Can you work these out from the model? Positions are in its coordinate system, mm. A direction names the side the tool comes from. Round coordinates to 2 decimals unless told otherwise and drop trailing zeros. Loops run counter-clockwise (first coordinate to the right, second up) from the corner with the lowest first, then second, coordinate; pieces in that order, holes last.
(1) I want a section at A-A on x = 0. Write out the boundary of the cut face in (y, z).
(2) I want a section at B-B on y = 12.5. Write out the boundary of the cut face in (x, z), plus the area to 3 significant figures.
(3) If I drill on line 1 along Y through (x, z) = (4.15, 0); line 2 along X through (y, z) = (8, 0); line 3 along X through (y, z) = (-12, -2.75), over which ranges is the centre line in solid material (lowest first)?
(4) Will these pins go through, and if not, where does the flat tip stop? pin 1 Ø0.8 at (x, z) = (0.5, -4) entering from -Y; pin 2 Ø5 at (x, z) = (3.5, 1.5) entering from +Y; pin 3 Ø2.5 at (y, z) = (-1, -2) entering from -X; pin 4 Ø1.2 at (x, z) = (-0.5, -4) entering from +Y.
(5) Thinking about a two-plate mould opening in Y: for faces 6 (the face through (-4, 12, 0)), 7 (the face through (0, -2, 2.5)), 8 (the face through (0, 2.964, 4)), which applies, released by +Y, released by -Y, zero draft, split by the parting line, or undercut?
(6) I want a section at C-C on z = -3. Write out the boundary of the cut face in (x, y), plus the area to 3 significant figures.
(7) Which directions (+Z, -Z, +X, -X, +Y, -Y) give clear straight access to the entire face, cutting with the end or side of a thin tool? Please do faces 1 (the face through (0, -2, -2.5)), 2 (the face through (4, 12, 0)), 3 (the face through (2.5, 0, 0)), 4 (the face through (0, 2.964, -4)), 5 (the face through (0, -7.5, -4)).
(8) I want a section at D-D on y = -2. Write out the boundary of the cut face in (x, z), plus the area to 3 significant figures.
from build123d import *

# Parameters (mm, degrees)
BOSS_EXTRUDE1_DEPTH      = 7.5
BOSS_EXTRUDE1_DEPTH_BACK = 7.5
SKETCH1_R                = 5
BOSS_EXTRUDE3_DEPTH      = 7.5
BOSS_EXTRUDE4_START      = 7.5
BOSS_EXTRUDE4_DEPTH      = 7.5
CUT_EXTRUDE2_DEPTH       = 24.58495283
CUT_EXTRUDE2_DEPTH_BACK  = 24.58495283
SKETCH5_W                = 5
SKETCH5_H                = 5
CUT_EXTRUDE4_DEPTH       = 18.5
CUT_EXTRUDE4_DEPTH_BACK  = 7.5
SKETCH14_W               = 0.500000016
SKETCH14_H               = 2.5
CUT_EXTRUDE5_DEPTH       = 7.5
CUT_EXTRUDE5_DEPTH_BACK  = 7.5
CUT_EXTRUDE8_DEPTH       = 7.5
CUT_EXTRUDE8_DEPTH_BACK  = 7.5
SKETCH17_W               = 5
SKETCH17_H               = 4.6


with BuildPart() as part:
    # Sketch1 → Boss-Extrude1 (new, two sides: drawn at the far end of the back side and taken through both)
    with BuildSketch(Plane(origin=(0, 0, 0), x_dir=(1, 0, 0), z_dir=(0, 1, 0)).offset(-BOSS_EXTRUDE1_DEPTH_BACK)):
        with Locations(Location((0, 0, 0), (0, 0, 270))):
            Circle(SKETCH1_R)
    extrude(amount=BOSS_EXTRUDE1_DEPTH + BOSS_EXTRUDE1_DEPTH_BACK)

    # Sketch3 → Boss-Extrude3 (add)
    with BuildSketch(Plane(origin=(0, 7.5, 0), x_dir=(1, 0, 0), z_dir=(0, 1, 0))):
        with BuildLine():
            Line((-2.5, 4.330127019), (-2.5, -4.330127019))
            ThreePointArc((-2.5, -4.330127019), (-5, 0), (-2.5, 4.330127019))
        make_face()
        with BuildLine():
            Line((2.5, 4.330127019), (2.5, -4.330127019))
            ThreePointArc((2.5, -4.330127019), (5, 0), (2.5, 4.330127019))
        make_face()
    extrude(amount=BOSS_EXTRUDE3_DEPTH)

    # Sketch4 → Boss-Extrude4 (add)
    with BuildSketch(Plane.XZ.offset(7.5).offset(BOSS_EXTRUDE4_START)):
        with BuildLine():
            Line((-2.5, 4.330127019), (-2.5, -4.330127019))
            ThreePointArc((-2.5, -4.330127019), (-5, 0), (-2.5, 4.330127019))
        make_face()
        with BuildLine():
            Line((2.5, 4.330127019), (2.5, -4.330127019))
            ThreePointArc((2.5, -4.330127019), (5, 0), (2.5, 4.330127019))
        make_face()
    extrude(amount=-BOSS_EXTRUDE4_DEPTH)

    # Sketch5 → Cut-Extrude2 (cut, two sides: drawn at the far end of the back side and taken through both)
    with BuildSketch(Plane.XZ.offset(7.5).offset(-CUT_EXTRUDE2_DEPTH_BACK)):
        Rectangle(SKETCH5_W, SKETCH5_H)
    extrude(amount=CUT_EXTRUDE2_DEPTH + CUT_EXTRUDE2_DEPTH_BACK, mode=Mode.SUBTRACT)

    # Sketch10 → Cut-Extrude4 (cut, two sides: drawn at the far end of the back side and taken through both)
    with BuildSketch(Plane(origin=(-2.5, 0, 0), x_dir=(0, 0, -1), z_dir=(1, 0, 0)).offset(-CUT_EXTRUDE4_DEPTH_BACK)):
        with BuildLine():
            Line((-4.33012702, 10.66987298), (-4.331858603, 15.169872647))
            Line((-4.331858603, 15.169872647), (4.328395437, 15.169872647))
            Line((4.328395437, 15.169872647), (4.33012702, 10.66987298))
            ThreePointArc((4.33012702, 10.66987298), (0, 15), (-4.33012702, 10.66987298))
        make_face()
    extrude(amount=CUT_EXTRUDE4_DEPTH + CUT_EXTRUDE4_DEPTH_BACK, mode=Mode.SUBTRACT)


with BuildPart() as cut_extrude4_piece_1:
    # of the separate pieces the step leaves, piece 1, a body of its own (cut_extrude4_pieces)
    add(part.part.solids().sort_by_distance((0, 0, 5))[0])

    # Sketch14 → 97 _0.03937008_ Diameter Hole1 (revolve, cut)
    with BuildSketch(Plane(origin=(2.5, 12.5, 0), x_dir=(0, 0, 1), z_dir=(0, 1, 0))):
        with Locations((0.250000008, 1.25)):
            Rectangle(SKETCH14_W, SKETCH14_H)
    revolve(axis=Axis((-3.85, 12.5, 0), (1, 0, 0)), mode=Mode.SUBTRACT)

    # Sketch15 → 97 _0.03937008_ Diameter Hole2 (revolve, cut)
    with BuildSketch(Plane(origin=(2.5, 12.5, 0), x_dir=(0, 0, -1), z_dir=(0, 1, 0))):
        Polygon((0, 0), (0, 10.300430319), (0.500000016, 10), (0.500000016, 0), align=None)
    revolve(axis=Axis((8.85, 12.5, 0), (-1, 0, 0)), mode=Mode.SUBTRACT)


with BuildPart() as cut_extrude4_piece_2:
    # of the separate pieces the step leaves, piece 2, a body of its own (cut_extrude4_pieces)
    add(part.part.solids().sort_by_distance((2.5, 15, -4.330127019))[0])


with BuildPart() as cut_extrude4_piece_3:
    # of the separate pieces the step leaves, piece 3, a body of its own (cut_extrude4_pieces)
    add(part.part.solids().sort_by_distance((-2.5, 15, -4.330127019))[0])


with BuildPart() as cut_extrude5_tool:
    # Sketch16 → Cut-Extrude5 (new, two sides: drawn at the far end of the back side and taken through both)
    with BuildSketch(Plane(origin=(-2.5, 0, 0), x_dir=(0, 0, -1), z_dir=(1, 0, 0)).offset(-CUT_EXTRUDE5_DEPTH_BACK)):
        with BuildLine():
            Line((5.450138396, 3.309889021), (7.392049741, 3.309889021))
            Line((7.392049741, 3.309889021), (7.392049741, 15))
            Line((7.392049741, 15), (0, 15))
            ThreePointArc((0, 15), (1.271548544, 14.652478641), (2.189584866, 13.70653144))
            ThreePointArc((2.189584866, 13.70653144), (3.387744198, 10.686815519), (3.795708462, 7.463799045))
            ThreePointArc((3.795708462, 7.463799045), (4.224533696, 5.228172349), (5.450138396, 3.309889021))
        make_face()
    extrude(amount=CUT_EXTRUDE5_DEPTH + CUT_EXTRUDE5_DEPTH_BACK)


with BuildPart() as cut_extrude4_piece_1_1:
    add(cut_extrude4_piece_1.part)

    # Cut-Extrude5: cut by cut_extrude5_tool
    add(cut_extrude5_tool.part, mode=Mode.SUBTRACT)

    # Sketch17 → Cut-Extrude8 (cut, two sides: drawn at the far end of the back side and taken through both)
    with BuildSketch(Plane.XY.offset(-CUT_EXTRUDE8_DEPTH_BACK)):
        with Locations((0, 5.263799045)):
            Rectangle(SKETCH17_W, SKETCH17_H)
    extrude(amount=CUT_EXTRUDE8_DEPTH + CUT_EXTRUDE8_DEPTH_BACK, mode=Mode.SUBTRACT)


with BuildPart() as cut_extrude4_piece_2_1:
    add(cut_extrude4_piece_2.part)

    # Cut-Extrude5: cut by cut_extrude5_tool
    add(cut_extrude5_tool.part, mode=Mode.SUBTRACT)


with BuildPart() as cut_extrude4_piece_3_1:
    add(cut_extrude4_piece_3.part)

    # Cut-Extrude5: cut by cut_extrude5_tool
    add(cut_extrude5_tool.part, mode=Mode.SUBTRACT)


solid = cut_extrude4_piece_1_1.part
Filled sheet:
1. outline: (-7.5, -5) - (2.96, -5) - (2.96, -2.5) - (-7.5, -2.5) - close; (-7.5, 2.5) - (2.96, 2.5) - (2.96, 5) - (-7.5, 5) - close
2. outline: (-4.97, -0.5) arc R5 ccw to (-4.16, -2.78) - (-2.5, -2.78) - (-2.5, -0.5) - close; (-4.97, 0.5) - (-2.5, 0.5) - (-2.5, 3.92) - (-3.1, 3.92) arc R5 ccw to start; (2.5, -2.78) - (4.16, -2.78) arc R5 ccw to (4.97, -0.5) - (2.5, -0.5) - close; (2.5, 0.5) - (4.97, 0.5) arc R5 ccw to (3.1, 3.92) - (2.5, 3.92) - close
2. area: 22.5 mm2
3. line 1: y = -15 to 12, 13 to 15
3. line 2: x = -5 to -2.5, 2.5 to 5
3. line 3: x = -4.18 to -2.5, 2.5 to 4.18
4. pin 1: stops at y = -7.5
4. pin 2: stops at y = 15
4. pin 3: stops at x = -4.94
4. pin 4: stops at y = 2.96
5. face 6: undercut
5. face 7: zero draft
5. face 8: released by +Y
6. outline: (-4, -15) - (-2.5, -15) - (-2.5, -7.5) - (2.5, -7.5) - (2.5, -15) - (4, -15) - (4, 11.93) - (2.5, 11.93) - (2.5, 2.96) - (-2.5, 2.96) - (-2.5, 11.93) - (-4, 11.93) - close
6. area: 133 mm2
7. face 1: +Y, -Y
7. face 2: +X, -X
7. face 3: none
7. face 4: +Z, -Z, +Y
7. face 5: +Z, -Z, -Y
8. outline: circle Ø10 at (0, 0); hole (-2.5, -2.5) - (2.5, -2.5) - (2.5, 2.5) - (-2.5, 2.5) - close
8. area: 53.5 mm2
